Read the model definition and answer for the solid it produces. Units are mm, in the model's axes. Face numbers are marked on the shaded views. A direction names the side the tool comes from. Give positions to 0.01 mm unless a question says otherwise; leave off trailing zeros. Order: outer loops, then holes, each group sorted by start corner. A loop starts at its lowest first (then second) coordinate and runs counter-clockwise, first axis right, second up. Notation, with made-up numbers: (40.5, 31) -> (47.5, 31) arc R13 cw to (47.5, 41) -> close; hole circle Ø7 at (-25, -13.5). An arc over 180 degrees is marked (long way). Use one line per item in the form item = value.
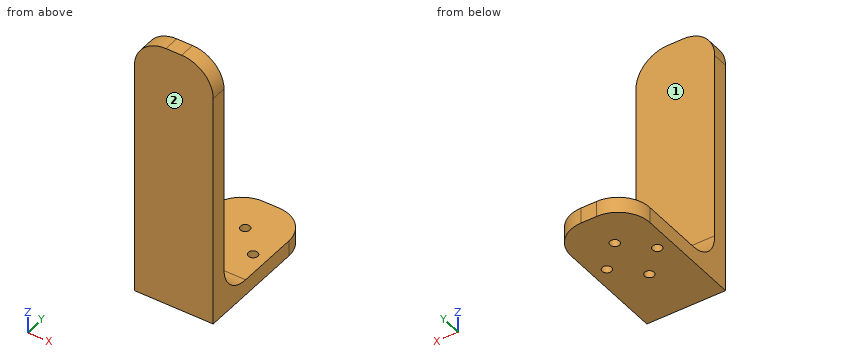
```python
from build123d import *

# Parameters (mm, degrees)
SKETCH_1_W      = 25
SKETCH_1_H      = 40
SKETCH_1_R      = 1.5
EXTRUDE_1_DEPTH = 5
SKETCH_2_W      = 25
SKETCH_2_H      = 85
EXTRUDE_2_DEPTH = 5
FILLET_1_R      = 10


with BuildPart() as part:
    # 草图1 → 凸台-拉伸1 (new body)
    with BuildSketch(Plane.XY):
        Rectangle(SKETCH_1_W, SKETCH_1_H)
        with Locations((0, 8)):
            Circle(SKETCH_1_R, mode=Mode.SUBTRACT)
        with Locations((8, 0)):
            Circle(SKETCH_1_R, mode=Mode.SUBTRACT)
        with Locations((0, -8)):
            Circle(SKETCH_1_R, mode=Mode.SUBTRACT)
        with Locations((-8, 0)):
            Circle(SKETCH_1_R, mode=Mode.SUBTRACT)
    extrude(amount=EXTRUDE_1_DEPTH)

    # 草图2 → 凸台-拉伸2 (add)
    with BuildSketch(Plane.XZ.offset(20)):
        with Locations((0, 42.5)):
            Rectangle(SKETCH_2_W, SKETCH_2_H)
    extrude(amount=EXTRUDE_2_DEPTH)

    # 圆角1
    fillet_1_edges = [part.edges().sort_by_distance(p)[0] for p in [
        (-12.5, -22.5, 85),
        (12.5, -22.5, 85),
        (-12.5, 20, 2.5),
        (12.5, 20, 2.5),
        (0, -20, 5),
    ]]
    fillet(fillet_1_edges, radius=FILLET_1_R)


solid = part.part
```
Item 1: The part is cut by section A-A on y = -8. Give the vertices of the cut face in (x, z), and give its area (3 significant figures).
Checks:
outline = (-12.5, 0) -> (-1.5, 0) -> (-1.5, 5) -> (-12.5, 5) -> close; (1.5, 0) -> (12.5, 0) -> (12.5, 5) -> (1.5, 5) -> close
area = 110 mm²
Item 2: Given pin 1 Ø5 at (x, z) = (0.5, 64) entering from +Y; pin 2 Ø2 at (x, y) = (-9.5, -11.5) entering from +Z; pin 3 Ø1 at (x, z) = (6, 8.5) entering from +Y, each flat-ended and moving along its own axis, determine where each tip first touches the part or whether it passes through.
Checks:
pin_1 = -20
pin_2 = 5.32
pin_3 = -17.14
Item 3: Straight lines are drawn through the part: L1, parallel to Y at x = 0, z = 3.7; L2, parallel to Y at x = -6.25, z = 36; L3, parallel to Z at x = -2.5, y = 16. For each, find the intervals that lie inside material, in ascending order. Write a range as from..to.
Checks:
L1 = -25..-9.5, -6.5..6.5, 9.5..20
L2 = -25..-20
L3 = 0..5
Item 4: Which of the six approach directions +Z, -Z, +X, -X, +Y, -Y give full straight-line access (tool end or side, diameter ignored) to the marked faces 1 and 2?
Checks:
face_1 = +Z, +X, -X, +Y
face_2 = +Z, -Z, +X, -X, -Y
Item 5: The part is cut by section B-B on x = 0. Give the vertices of the cut face in (y, z), and give its area (3 significant figures).
Checks:
outline = (-25, 0) -> (-9.5, 0) -> (-9.5, 5) -> (-10, 5) arc R10 cw to (-20, 15) -> (-20, 85) -> (-25, 85) -> close; (-6.5, 0) -> (6.5, 0) -> (6.5, 5) -> (-6.5, 5) -> close; (9.5, 0) -> (20, 0) -> (20, 5) -> (9.5, 5) -> close
area = 616 mm²
Item 6: The part is cut by section C-C on y = 0. Give the vertices of the cut face in (x, z), and give its area (3 significant figures).
Checks:
outline = (-12.5, 0) -> (-9.5, 0) -> (-9.5, 5) -> (-12.5, 5) -> close; (-6.5, 0) -> (6.5, 0) -> (6.5, 5) -> (-6.5, 5) -> close; (9.5, 0) -> (12.5, 0) -> (12.5, 5) -> (9.5, 5) -> close
area = 95.0 mm²
Item 7: The part is cut by section D-D on x = 8. Give the vertices of the cut face in (y, z), and give its area (3 significant figures).
Checks:
outline = (-25, 0) -> (-1.5, 0) -> (-1.5, 5) -> (-10, 5) arc R10 cw to (-20, 15) -> (-20, 83.35) -> (-25, 83.35) -> close; (1.5, 0) -> (18.35, 0) -> (18.35, 5) -> (1.5, 5) -> close
area = 615 mm²
